Check sheet for the modelled part. Datum: model origin and axes. Units: mm. A direction names the side the tool comes from. Round coordinates to 2 decimals unless told otherwise and drop trailing zeros. Loops run counter-clockwise (first coordinate to the right, second up) from the corner with the lowest first, then second, coordinate; pieces in that order, holes last. Notation, with made-up numbers: (59.25, 66) -> (112.25, 66) arc R24 ccw to (112.25, 100) -> close; hole circle Ø2 at (-3, 7.5). An arc over 180 degrees is marked (long way). One line per question, with ' | ' between items.
```python
from build123d import *

# Parameters (mm, degrees)
SKETCH_1_W          = 90.5
SKETCH_1_H          = 97
EXTRUDE_1_DEPTH     = 2
SKETCH_2_W          = 104.525
SKETCH_2_H          = 124
SKETCH_2_R          = 1.6
EXTRUDE_2_DEPTH     = 2.5
SKETCH_3_W          = 88.5
SKETCH_3_H          = 17
EXTRUDE_3_DEPTH     = 2
SKETCH_4_W          = 1
SKETCH_4_H          = 5
CUT_EXTRUDE_1_DEPTH = 2
CUT_EXTRUDE_2_DEPTH = 150.601890446
SKETCH_6_W          = 45
SKETCH_6_H          = 25
CUT_EXTRUDE_3_DEPTH = 1.7
CUT_EXTRUDE_4_REACH = 146.972
SKETCH_7_R          = 1.6
CHAMFER_1_SIZE      = 2
CUT_EXTRUDE_5_REACH = 147.014
SKETCH_8_R          = 2.05
CUT_EXTRUDE_6_REACH = 147.014
SKETCH_9_R          = 10
CUT_EXTRUDE_7_DEPTH = 0.8
CUT_EXTRUDE_8_REACH = 151.602
SKETCH_11_W         = 6.5
SKETCH_11_H         = 2.5
CHAMFER_2_SIZE      = 2
SKETCH_12_W         = 104.525
SKETCH_12_H         = 9.5
EXTRUDE_4_DEPTH     = 1
SKETCH_13_W         = 2
SKETCH_13_H         = 14.5
EXTRUDE_5_DEPTH     = 0.5
SKETCH_14_W         = 1.5
SKETCH_14_H         = 9
SKETCH_14_W_2       = 1
EXTRUDE_6_DEPTH     = 0.5
SKETCH_15_W         = 88.5
SKETCH_15_H         = 2.828427125
EXTRUDE_7_DEPTH     = 2
CUT_EXTRUDE_9_DEPTH = 0.5


with BuildPart() as part:
    # 草图1 → 凸台-拉伸1 (new body)
    with BuildSketch(Plane(origin=(0, 0, 0), x_dir=(1, 0, 0), z_dir=(0, 1, 0))):
        with Locations((45.25, 48.5)):
            Rectangle(SKETCH_1_W, SKETCH_1_H)
    extrude(amount=EXTRUDE_1_DEPTH)

    # 草图2 → 凸台-拉伸2 (add)
    with BuildSketch(Plane.XZ):
        with Locations((45.5125, -45)):
            Rectangle(SKETCH_2_W, SKETCH_2_H)
        with Locations(Location((21.25, -102, 0), (0, 0, 270))):
            Circle(SKETCH_2_R, mode=Mode.SUBTRACT)
        with Locations(Location((69.25, -102, 0), (0, 0, 270))):
            Circle(SKETCH_2_R, mode=Mode.SUBTRACT)
        with Locations(Location((-3.25, -89, 0), (0, 0, 270))):
            Circle(SKETCH_2_R, mode=Mode.SUBTRACT)
        with Locations(Location((94.275, -90.75, 0), (0, 0, 270))):
            Circle(SKETCH_2_R, mode=Mode.SUBTRACT)
        with Locations(Location((-3.25, -13, 0), (0, 0, 270))):
            Circle(SKETCH_2_R, mode=Mode.SUBTRACT)
        with Locations(Location((-3.25, -51, 0), (0, 0, 270))):
            Circle(SKETCH_2_R, mode=Mode.SUBTRACT)
        with Locations(Location((94.275, -9.75, 0), (0, 0, 270))):
            Circle(SKETCH_2_R, mode=Mode.SUBTRACT)
        with Locations(Location((94.275, -45.75, 0), (0, 0, 270))):
            Circle(SKETCH_2_R, mode=Mode.SUBTRACT)
    extrude(amount=EXTRUDE_2_DEPTH)

    # 草图3 → 凸台-拉伸3 (add)
    with BuildSketch(Plane(origin=(0, 0, 0), x_dir=(1, 0, 0), z_dir=(0, 1, 0))):
        with Locations((45.25, -8.5)):
            Rectangle(SKETCH_3_W, SKETCH_3_H)
    extrude(amount=EXTRUDE_3_DEPTH)

    # 草图4 → 切除-拉伸1 (cut)
    with BuildSketch(Plane(origin=(0, 0, 0), x_dir=(1, 0, 0), z_dir=(0, 1, 0))):
        with Locations((0.5, 2.5)):
            Rectangle(SKETCH_4_W, SKETCH_4_H)
        with Locations((90, 2.5)):
            Rectangle(SKETCH_4_W, SKETCH_4_H)
    extrude(amount=CUT_EXTRUDE_1_DEPTH, mode=Mode.SUBTRACT)

    # 草图5 → 切除-拉伸2 (cut, through all)
    with BuildSketch(Plane(origin=(97.775, 0, 0), x_dir=(0, 0, -1), z_dir=(1, 0, 0))):
        Polygon((-8.5, -2.5), (-8.5, 0), (-9.5, 0), (-11.5, 2), (-17, 2), (-17, -2.5), align=None)
    extrude(amount=-CUT_EXTRUDE_2_DEPTH, mode=Mode.SUBTRACT)

    # 草图6 → 切除-拉伸3 (cut)
    with BuildSketch(Plane(origin=(0, 2, 0), x_dir=(1, 0, 0), z_dir=(0, 1, 0))):
        with Locations((45.5125, 34.5)):
            Rectangle(SKETCH_6_W, SKETCH_6_H)
    extrude(amount=-CUT_EXTRUDE_3_DEPTH, mode=Mode.SUBTRACT)

    # 草图7 → 切除-拉伸4 (cut, up to next)
    with BuildSketch(Plane(origin=(0, 0.3, 0), x_dir=(1, 0, 0), z_dir=(0, 1, 0)), mode=Mode.PRIVATE) as cut_extrude_4_sk1:
        with Locations(Location((30.5125, 27.5, 0), (0, 0, 270))):
            Circle(SKETCH_7_R)
    cut_extrude_4_tool1 = extrude(cut_extrude_4_sk1.sketch, amount=-CUT_EXTRUDE_4_REACH, mode=Mode.PRIVATE) & part.part
    # 草图7 → 切除-拉伸4 (cut, up to next)
    with BuildSketch(Plane(origin=(0, 0.3, 0), x_dir=(1, 0, 0), z_dir=(0, 1, 0)), mode=Mode.PRIVATE) as cut_extrude_4_sk2:
        with Locations(Location((60.5125, 27.5, 0), (0, 0, 270))):
            Circle(SKETCH_7_R)
    cut_extrude_4_tool2 = extrude(cut_extrude_4_sk2.sketch, amount=-CUT_EXTRUDE_4_REACH, mode=Mode.PRIVATE) & part.part
    add(cut_extrude_4_tool1.solids().sort_by_distance((30.5125, 0.3, -27.5))[0], mode=Mode.SUBTRACT)
    add(cut_extrude_4_tool2.solids().sort_by_distance((60.5125, 0.3, -27.5))[0], mode=Mode.SUBTRACT)

    # 倒角1
    # the kernel refuses this chamfer: 2 mm, written as the material it adds along each edge
    # the kernel refuses this chamfer: 2 mm, written as the material it takes off along each edge
    with BuildSketch(Plane(origin=(23.0125, 2, -47), x_dir=(0, 0.027495876610586296, -0.9996219169112968), z_dir=(1, 0, 0))) as chamfer_1_2_piece_1_section:
        Polygon((CHAMFER_1_SIZE * 0.999621916911, -CHAMFER_1_SIZE * 0.0274958766106), (-CHAMFER_1_SIZE * 0.0274958766106, -CHAMFER_1_SIZE * 0.999621916911), (0, 0), align=None)
    chamfer_1_2_piece_1 = extrude(amount=45, mode=Mode.PRIVATE)
    chamfer_1_2_piece_1 = split(chamfer_1_2_piece_1, bisect_by=Plane(origin=(45.5125, 0.3, -47.679710145), z_dir=(0, 1, 0)), keep=Keep.TOP, mode=Mode.PRIVATE)
    add(chamfer_1_2_piece_1, mode=Mode.SUBTRACT)

    # 草图8 → 切除-拉伸5 (cut, up to next)
    with BuildSketch(Plane(origin=(0, 2, 0), x_dir=(1, 0, 0), z_dir=(0, 1, 0)), mode=Mode.PRIVATE) as cut_extrude_5_sk1:
        with Locations(Location((20.5125, 77, 0), (0, 0, 270))):
            Circle(SKETCH_8_R)
    cut_extrude_5_tool1 = extrude(cut_extrude_5_sk1.sketch, amount=-CUT_EXTRUDE_5_REACH, mode=Mode.PRIVATE) & part.part
    # 草图8 → 切除-拉伸5 (cut, up to next)
    with BuildSketch(Plane(origin=(0, 2, 0), x_dir=(1, 0, 0), z_dir=(0, 1, 0)), mode=Mode.PRIVATE) as cut_extrude_5_sk2:
        with Locations(Location((70.5125, 77, 0), (0, 0, 270))):
            Circle(SKETCH_8_R)
    cut_extrude_5_tool2 = extrude(cut_extrude_5_sk2.sketch, amount=-CUT_EXTRUDE_5_REACH, mode=Mode.PRIVATE) & part.part
    # 草图8 → 切除-拉伸5 (cut, up to next)
    with BuildSketch(Plane(origin=(0, 2, 0), x_dir=(1, 0, 0), z_dir=(0, 1, 0)), mode=Mode.PRIVATE) as cut_extrude_5_sk3:
        with Locations(Location((15.5125, 32, 0), (0, 0, 270))):
            Circle(SKETCH_8_R)
    cut_extrude_5_tool3 = extrude(cut_extrude_5_sk3.sketch, amount=-CUT_EXTRUDE_5_REACH, mode=Mode.PRIVATE) & part.part
    # 草图8 → 切除-拉伸5 (cut, up to next)
    with BuildSketch(Plane(origin=(0, 2, 0), x_dir=(1, 0, 0), z_dir=(0, 1, 0)), mode=Mode.PRIVATE) as cut_extrude_5_sk4:
        with Locations(Location((75.5125, 32, 0), (0, 0, 270))):
            Circle(SKETCH_8_R)
    cut_extrude_5_tool4 = extrude(cut_extrude_5_sk4.sketch, amount=-CUT_EXTRUDE_5_REACH, mode=Mode.PRIVATE) & part.part
    add(cut_extrude_5_tool1.solids().sort_by_distance((20.5125, 2, -77))[0], mode=Mode.SUBTRACT)
    add(cut_extrude_5_tool2.solids().sort_by_distance((70.5125, 2, -77))[0], mode=Mode.SUBTRACT)
    add(cut_extrude_5_tool3.solids().sort_by_distance((15.5125, 2, -32))[0], mode=Mode.SUBTRACT)
    add(cut_extrude_5_tool4.solids().sort_by_distance((75.5125, 2, -32))[0], mode=Mode.SUBTRACT)

    # 草图9 → 切除-拉伸6 (cut, up to next)
    with BuildSketch(Plane(origin=(0, 2, 0), x_dir=(1, 0, 0), z_dir=(0, 1, 0)), mode=Mode.PRIVATE) as cut_extrude_6_sk1:
        with Locations(Location((45.5125, 55, 0), (0, 0, 230.353888853))):
            Circle(SKETCH_9_R)
    cut_extrude_6_tool1 = extrude(cut_extrude_6_sk1.sketch, amount=-CUT_EXTRUDE_6_REACH, mode=Mode.PRIVATE) & part.part
    add(cut_extrude_6_tool1.solids().sort_by_distance((45.5125, 2, -55))[0], mode=Mode.SUBTRACT)

    # 草图10 → 切除-拉伸7 (cut)
    with BuildSketch(Plane.XZ.offset(2.5)):
        Polygon((27.7625, -25.91228676), (27.7625, -29.08771324), (30.5125, -30.675426481), (33.2625, -29.08771324), (33.2625, -25.91228676), (30.5125, -24.324573519), align=None)
        Polygon((57.7625, -25.91228676), (57.7625, -29.08771324), (60.5125, -30.675426481), (63.2625, -29.08771324), (63.2625, -25.91228676), (60.5125, -24.324573519), align=None)
    extrude(amount=-CUT_EXTRUDE_7_DEPTH, mode=Mode.SUBTRACT)

    # 草图11 → 切除-拉伸8 (cut, up to next)
    with BuildSketch(Plane(origin=(97.775, 0, 0), x_dir=(0, 0, -1), z_dir=(1, 0, 0)), mode=Mode.PRIVATE) as cut_extrude_8_sk1:
        with Locations((-5.25, -1.25)):
            Rectangle(SKETCH_11_W, SKETCH_11_H)
    cut_extrude_8_tool1 = extrude(cut_extrude_8_sk1.sketch, amount=-CUT_EXTRUDE_8_REACH, mode=Mode.PRIVATE) & part.part
    add(cut_extrude_8_tool1.solids().sort_by_distance((97.775, -1.25, 5.25))[0], mode=Mode.SUBTRACT)

    # 倒角2
    chamfer_2_edges = [part.edges().sort_by_distance(p)[0] for p in [
        (45.5125, -2.5, 2),
    ]]
    chamfer(chamfer_2_edges, length=CHAMFER_2_SIZE)

    # 草图12 → 凸台-拉伸4 (add)
    with BuildSketch(Plane.XZ):
        with Locations((45.5125, 4.75)):
            Rectangle(SKETCH_12_W, SKETCH_12_H)
    extrude(amount=EXTRUDE_4_DEPTH)

    # 草图13 → 凸台-拉伸5 (add)
    with BuildSketch(Plane(origin=(0, 0, 0), x_dir=(1, 0, 0), z_dir=(0, 1, 0))):
        with Locations((0, -2.25)):
            Rectangle(SKETCH_13_W, SKETCH_13_H)
        with Locations((90.5, -2.25)):
            Rectangle(SKETCH_13_W, SKETCH_13_H)
    extrude(amount=EXTRUDE_5_DEPTH)

    # 草图14 → 凸台-拉伸6 (add)
    with BuildSketch(Plane(origin=(0, 0, 0), x_dir=(1, 0, 0), z_dir=(0, 1, 0))):
        with Locations((92.25, -5)):
            Rectangle(SKETCH_14_W, SKETCH_14_H)
        with Locations((-1.5, -5)):
            Rectangle(SKETCH_14_W_2, SKETCH_14_H)
    extrude(amount=EXTRUDE_6_DEPTH)

    # 草图15 → 凸台-拉伸7 (add, along a direction that is not the sketch's normal)
    with BuildSketch(Plane(origin=(0, -4.75, 4.75), x_dir=(1, 0, 0), z_dir=(0, -0.7071067811865501, 0.7071067811865449))):
        with Locations((45.25, 8.131727983)):
            Rectangle(SKETCH_15_W, SKETCH_15_H)
    extrude(amount=EXTRUDE_7_DEPTH, dir=(0, 0, 1))

    # 草图16 → 切除-拉伸9 (cut)
    with BuildSketch(Plane(origin=(0, 2, 0), x_dir=(1, 0, 0), z_dir=(0, 1, 0))):
        Polygon((1, 5), (1, -13.5), (89.5, -13.5), (89.5, 5), (90.5, 5), (90.5, 97), (0, 97), (0, 5), align=None)
    extrude(amount=-CUT_EXTRUDE_9_DEPTH, mode=Mode.SUBTRACT)


solid = part.part
```
(1) Scan lines: probe 1 along X at (y, z) = (0.55, -77); probe 2 along X at (y, z) = (0.4, -32); probe 3 along Z at (x, y) = (70.5, -2.25). Record each from-to range of solid material in increasing order.
Answer:
probe 1: x = 0 to 18.46, 22.56 to 68.46, 72.56 to 90.5 | probe 2: x = 0 to 13.46, 17.56 to 23.01, 68.01 to 73.46, 77.56 to 90.5 | probe 3: z = -107 to -103, -101 to -79.05, -74.95 to 0.25
(2) Go/stop test with flat-tipped pins: pin 1 (1.9 mm diameter, centred on x = 60.51, z = -27.5, fed in from +Y); pin 2 (0.6 mm diameter, centred on x = 27.5, z = 11, fed in from -Y); pin 3 (4 mm diameter, centred on x = -3.25, z = -51, fed in from +Y); pin 4 (1.2 mm diameter, centred on x = 65.5, y = 1, fed in from -Z). Record where each tip stops, or that it passes through.
Answer:
pin 1: passes through | pin 2: stops at y = 0 | pin 3: stops at y = 0 | pin 4: stops at z = -97
(3) Set-up check for faces 1 (the face through (45, 0.3, -35)), 2 (the face through (45, -1, 6)), 3 (the face through (91, 0.5, 4)), 4 (the face through (-1, 0.5, 2)): record each of +Z, -Z, +X, -X, +Y, -Y from which the full face is reachable in a straight line by a thin tool's end or side.
Answer:
face 1: +Y | face 2: +Z, +X, -X, -Y | face 3: +Z, +X, +Y | face 4: +Z, -X, +Y
(4) Sectioned sample at A-A, the plane z = -77. Count the separate pieces of the cut face and the enclosed holes in it, and give its area (3 significant figures).
Answer:
separate pieces: 3 | enclosed holes: 0 | area: 364 mm2
(5) Mould release check, pull along Z, two halves, no side actions. Record for faces 5 (the face through (35, 1.5, -55)), 6 (the face through (32, -1.7, -29)): +Z half, -Z half, draft (parallel to the pull), parting line (faces both ways), or undercut.
Answer:
face 5: draft | face 6: undercut
(6) Sectioned sample at C-C, the plane x = 10. Record the cut outline in (y, z).
Answer:
outline: (-2.5, -107) -> (0, -107) -> (0, -97) -> (1.5, -97) -> (1.5, 13) -> (0, 11.5) -> (0, 9.5) -> (-1, 9.5) -> (-1, 1.5) -> (-2.5, 0) -> close
(7) Sectioned sample at B-B, the plane z = -13. Record the cut outline in (x, y) (3 decimals).
Answer:
outline: (-6.75, -2.5) -> (-4.85, -2.5) -> (-4.85, 0) -> (-6.75, 0) -> close; (-1.65, -2.5) -> (97.775, -2.5) -> (97.775, 0) -> (90.5, 0) -> (90.5, 1.5) -> (0, 1.5) -> (0, 0) -> (-1.65, 0) -> close
